For this review, take the finished solid that the model builds, in its own axes (mm). A direction names the side the tool comes from. Give positions to 0.01 mm unless a question says otherwise; leave off trailing zeros. Order: outer loops, then holes, each group sorted by start corner. A loop starts at its lowest first (then second) coordinate and runs counter-clockwise, first axis right, second up.
from build123d import *

# Parameters (mm, degrees)
EXTRUDE_START       = -75
EXTRUDE_1_DEPTH     = 150
SKETCH_2_R          = 5.5
CUT_EXTRUDE_1_DEPTH = 6
SKETCH_3_R          = 3.3
CUT_EXTRUDE_2_DEPTH = 82.547532152


# Read off the part's stored shape, not the designer's step: 凸台-拉伸1
with BuildPart() as part:
    # 凸台-拉伸1 outline → 凸台-拉伸1 (new body)
    with BuildSketch(Plane(origin=(0, 0, 0), x_dir=(0, 0, -1), z_dir=(1, 0, 0)).offset(EXTRUDE_START)):
        Polygon((20, 0), (20, 10), (10, 10), (10, 25), (-10, 25), (-10, 10), (-20, 10), (-20, 0), align=None)
    extrude(amount=EXTRUDE_1_DEPTH)

    # 草图2 → 切除-拉伸1 (cut)
    with BuildSketch(Plane(origin=(0, 25, 0), x_dir=(1, 0, 0), z_dir=(0, 1, 0))):
        with Locations(Location((-60, 0, 0), (0, 0, 270))):
            Circle(SKETCH_2_R)
        with Locations(Location((0, 0, 0), (0, 0, 270))):
            Circle(SKETCH_2_R)
        with Locations(Location((60, 0, 0), (0, 0, 270))):
            Circle(SKETCH_2_R)
    extrude(amount=-CUT_EXTRUDE_1_DEPTH, mode=Mode.SUBTRACT)

    # 草图3 → 切除-拉伸2 (cut, through all)
    with BuildSketch(Plane(origin=(0, 25, 0), x_dir=(1, 0, 0), z_dir=(0, 1, 0))):
        with Locations(Location((-60, 0, 0), (0, 0, 270))):
            Circle(SKETCH_3_R)
        with Locations(Location((0, 0, 0), (0, 0, 270))):
            Circle(SKETCH_3_R)
        with Locations(Location((60, 0, 0), (0, 0, 270))):
            Circle(SKETCH_3_R)
    extrude(amount=-CUT_EXTRUDE_2_DEPTH, mode=Mode.SUBTRACT)


solid = part.part
1) Draft analysis for pull direction Z (two halves, no side actions). For faces 5 (the face through (-1, 18, 10)), 6 (the face through (56, 19, 0)), 7 (the face through (75, 10, 0)), state which applies: +Z half, -Z half, draft (parallel to the pull), parting line (faces both ways), or undercut.
Answer sheet:
face 5: +Z half
face 6: undercut
face 7: draft
2) Tool access review of faces 1 (the face through (-1, 17, -10)), 2 (the face through (-75, 10, 0)), 3 (the face through (65.453, 22.042, -0.716)), 4 (the face through (-1, 10, 15)): name each direction out of +Z, -Z, +X, -X, +Y, -Y from which nothing blocks a thin tool from reaching the whole face with its end or side.
Answer sheet:
face 1: -Z, +X, -X, +Y
face 2: +Z, -Z, -X, +Y, -Y
face 3: +Y
face 4: +Z, +X, -X, +Y
3) Clearance check with flat-ended pins moving along their axes: pin 1 (4 mm diameter, centred on x = -59.5, y = 13, fed in from -Z); pin 2 (3 mm diameter, centred on x = -37.5, z = 15.5, fed in from +Y); pin 3 (6 mm diameter, centred on x = -19.5, y = 21, fed in from +Z); pin 4 (12.5 mm diameter, centred on x = 60, z = 0, fed in from +Y). State where each tip first meets the part, or that it passes through.
Answer sheet:
pin 1: stops at z = -10
pin 2: stops at y = 10
pin 3: stops at z = 10
pin 4: stops at y = 25
4) We need section D-D on x = 15. Give the boundary of the cut face in (y, z).
Answer sheet:
outline: (0, -20) - (10, -20) - (10, -10) - (25, -10) - (25, 10) - (10, 10) - (10, 20) - (0, 20) - close
5) We need section B-B on y = 5.75. Give the boundary of the cut face in (x, z).
Answer sheet:
outline: (-75, -20) - (75, -20) - (75, 20) - (-75, 20) - close; hole circle Ø6.6 at (-60, 0); hole circle Ø6.6 at (0, 0); hole circle Ø6.6 at (60, 0)
6) We need section C-C on z = 0. Give the boundary of the cut face in (x, y).
Answer sheet:
outline: (-75, 0) - (-63.3, 0) - (-63.3, 19) - (-65.5, 19) - (-65.5, 25) - (-75, 25) - close; (-56.7, 0) - (-3.3, 0) - (-3.3, 19) - (-5.5, 19) - (-5.5, 25) - (-54.5, 25) - (-54.5, 19) - (-56.7, 19) - close; (3.3, 0) - (56.7, 0) - (56.7, 19) - (54.5, 19) - (54.5, 25) - (5.5, 25) - (5.5, 19) - (3.3, 19) - close; (63.3, 0) - (75, 0) - (75, 25) - (65.5, 25) - (65.5, 19) - (63.3, 19) - close
7) To check wall thickness, follow line 1 (X direction, y = 10.5, z = 0); line 2 (X direction, y = 22.15, z = 0); line 3 (Z direction, x = -14, y = 19.5). State the ranges of each line that lie inside material, in increasing order.
Answer sheet:
line 1: x = -75 to -63.3, -56.7 to -3.3, 3.3 to 56.7, 63.3 to 75
line 2: x = -75 to -65.5, -54.5 to -5.5, 5.5 to 54.5, 65.5 to 75
line 3: z = -10 to 10
8) We need section A-A on x = -60. Give the boundary of the cut face in (y, z), then the cut area to 3 significant figures.
Answer sheet:
outline: (0, -20) - (10, -20) - (10, -10) - (25, -10) - (25, -5.5) - (19, -5.5) - (19, -3.3) - (0, -3.3) - close; (0, 3.3) - (19, 3.3) - (19, 5.5) - (25, 5.5) - (25, 10) - (10, 10) - (10, 20) - (0, 20) - close
area: 509 mm2
